Part model, mm, in its own coordinate system. A direction names the side the tool comes from. Round coordinates to 2 decimals unless told otherwise and drop trailing zeros. Order: outer loops, then holes, each group sorted by start corner. A loop starts at its lowest first (then second) coordinate and runs counter-clockwise, first axis right, second up. Notation, with made-up numbers: (4, -12.5) -> (22, -12.5) arc R14 cw to (22, -8.5) -> close; hole circle Ø10 at (89, 19.25). An arc over 180 degrees is marked (long way). Use CSV: the item, a comma, the result in double quotes.
```python
from build123d import *

# Parameters (mm, degrees)
SKETCH_1_R          = 2
EXTRUDE_1_DEPTH     = 30
SKETCH_2_R          = 3
SKETCH_2_W          = 30
SKETCH_2_H          = 11
CUT_EXTRUDE_1_DEPTH = 44.647021662
CHAMFER_1_SIZE      = 3


with BuildPart() as part:
    # 草图1 → 凸台-拉伸1 (new, symmetric)
    with BuildSketch(Plane(origin=(0, 0, 0), x_dir=(0, 0, -1), z_dir=(1, 0, 0))):
        with BuildLine():
            Line((0, 0), (30, 0))
            Line((30, 0), (30, 4))
            Line((30, 4), (5, 4))
            ThreePointArc((5, 4), (-3.201562119, 9.126952648), (0, 0))
        make_face()
        with Locations((0, 5.125)):
            Circle(SKETCH_1_R, mode=Mode.SUBTRACT)
    extrude(amount=EXTRUDE_1_DEPTH, both=True)

    # 草图2 → 切除-拉伸1 (cut, through all)
    with BuildSketch(Plane(origin=(0, 0, 0), x_dir=(1, 0, 0), z_dir=(0, 1, 0))):
        with Locations(Location((-17, 18.5, 0), (0, 0, 90))):
            Circle(SKETCH_2_R)
        with Locations(Location((17, 18.5, 0), (0, 0, 90))):
            Circle(SKETCH_2_R)
        with Locations((0, 0.375)):
            Rectangle(SKETCH_2_W, SKETCH_2_H)
    extrude(amount=CUT_EXTRUDE_1_DEPTH, mode=Mode.SUBTRACT)

    # 倒角1
    chamfer_1_edges = [part.edges().sort_by_distance(p)[0] for p in [
        (0, 4, -5.875),
        (17, 4, -15.5),
        (-17, 4, -15.5),
        (0, 4, -30),
    ]]
    chamfer(chamfer_1_edges, length=CHAMFER_1_SIZE)


solid = part.part
```
(1) Probe probe 1 along X at (y, z) = (0.6, -18.5); probe 2 along X at (y, z) = (3.75, -5); probe 3 along Y at (x, z) = (19.25, 0) (3 decimals). List the from-to ranges inside material, lowest first. Write a range as [from, to].
Reply:
probe 1,"[-30, -20], [-14, 14], [20, 30]"
probe 2,"[-30, -15], [15, 30]"
probe 3,"[0, 3.125], [7.125, 10.25]"
(2) Cut at A-A, the plane x = 17. Give the cut face in (y, z) (3 decimals).
Reply:
outline,"(0, -30) -> (1, -30) -> (4, -27) -> (4, -24.5) -> (1, -21.5) -> (0, -21.5) -> close; (0, -15.5) -> (1, -15.5) -> (4, -12.5) -> (4, -5) arc R5.125 ccw (long way) to (0, 0) -> close; hole circle Ø4 at (5.125, 0)"
(3) Cut at B-B, the plane z = -18.5. Give the cut face in (x, y).
Reply:
outline,"(-30, 0) -> (-20, 0) -> (-20, 1) -> (-23, 4) -> (-30, 4) -> close; (-14, 0) -> (14, 0) -> (14, 1) -> (11, 4) -> (-11, 4) -> (-14, 1) -> close; (20, 0) -> (30, 0) -> (30, 4) -> (23, 4) -> (20, 1) -> close"
(4) Drop a flat-ended pin along its axis: P1, Ø6.5, axis at x = -12.5, z = -14.5, coming from the +Y side. Give the stop position or say it passes through.
Reply:
P1,"y = 4"
(5) Which spindle directions (+Z, -Z, +X, -X, +Y, -Y) get a long thin tool onto all of the face, cutting with end or side? Do faces 5 (the face through (0.21, 2.479, -7.354)), 6 (the face through (0, 2, -29)). Say none if no direction does.
Reply:
face 5,"+Z, +Y"
face 6,"-Z, +X, -X, +Y"
(6) Cut at D-D, the plane y = 6.25. Give the cut face in (x, z), then the cut area to 3 significant figures.
Reply:
outline,"(-30, -5) -> (-15, -5) -> (-15, -1.65) -> (-30, -1.65) -> close; (-30, 1.65) -> (-15, 1.65) -> (-15, 5) -> (-30, 5) -> close; (15, -5) -> (30, -5) -> (30, -1.65) -> (15, -1.65) -> close; (15, 1.65) -> (30, 1.65) -> (30, 5) -> (15, 5) -> close"
area,"201 mm2"
(7) Pull direction X, two halves, no side cores. Call faces 1 (the face through (0, 4, -16)), 2 (the face through (-30, 3, -8)), 3 (the face through (18.8, 0.5, -16.1)), 4 (the face through (15, 4, -2)): released by +X, released by -X, zero draft, split by the parting line, or undercut.
Reply:
face 1,"zero draft"
face 2,"released by -X"
face 3,"undercut"
face 4,"undercut"
(8) Cut at C-C, the plane y = 2. Give the cut face in (x, z) (3 decimals), then the cut area to 3 significant figures.
Reply:
outline,"(-30, -29) -> (30, -29) -> (30, 4.062) -> (15, 4.062) -> (15, -6.875) -> (-15, -6.875) -> (-15, 4.062) -> (-30, 4.062) -> close; hole circle Ø8 at (-17, -18.5); hole circle Ø8 at (17, -18.5)"
area,"1,560 mm2"
